from build123d import *

# Parameters (mm, degrees)
EXTRUDE_THIN1_DEPTH   = 6
FILLET1_RADIUS        = 3
FILLET1_LENGTH        = 0.5
F_2_0MM_DOWEL_HOLE1_D = 2


with BuildPart() as part:
    # Sketch1 → Extrude-Thin1 (new body)
    with BuildSketch(Plane.XY):
        Polygon((0, 0), (-6, 0), (-36, 2), (-47.132818026, -3), (-47.337667505, -2.543889606), (-36.091128385, 2.507185105), (-5.983351811, 0.5), (0, 0.5), align=None)
    extrude(amount=EXTRUDE_THIN1_DEPTH)

    # Fillet1: full round fillet: the end face becomes a half cylinder, R = half its width
    fillet1_face = Plane((0, 0.25, 3), x_dir=(0, -1, 0), z_dir=(1, 0, 0))  # on the end face: x along it, z out of the body
    fillet1_slab = fillet1_face.offset(-FILLET1_RADIUS / 2) * Box(FILLET1_LENGTH, 2 * FILLET1_RADIUS, FILLET1_RADIUS, mode=Mode.PRIVATE)  # the body's end, R deep
    fillet1_round = Plane((-3, 0.25, 3), x_dir=(1, 0, 0), z_dir=(0, -1, 0)) * Cylinder(FILLET1_RADIUS, FILLET1_LENGTH, mode=Mode.PRIVATE)  # its axis R under the face
    add(fillet1_slab - fillet1_round, mode=Mode.SUBTRACT)

    # Ø2.0mm Dowel Hole1 (through all)
    with Locations(Plane(origin=(0, 0.5, 0), x_dir=(1, 0, 0), z_dir=(0, 1, 0))):
        with Locations((-3, -3)):
            Hole(F_2_0MM_DOWEL_HOLE1_D / 2)


solid = part.part
Can you work these out from the model? Positions are in its coordinate system, mm. A direction names the side the tool comes from. Give positions to 0.01 mm unless a question says otherwise; leave off trailing zeros. Write each loop counter-clockwise with the first axis right and the second up, starting at its lowest first coordinate (ties: lowest second). Pieces come first, ordered by that corner, then holes. Notation, with made-up numbers: (87, 16) -> (128, 16) arc R25 cw to (128, 47) -> close; hole circle Ø2 at (89, 4). An arc over 180 degrees is marked (long way). Answer as a JSON object with one key per item and string values. Group by question number.
Item 1: Please list where these lines run through material, in increasing order: line 1 (Z direction, x = -3, y = 0.1); line 2 (Y direction, x = -21, z = 4.95); line 3 (Y direction, x = -15.5, z = 3.4). Write a range as [from, to].
Item 2: We'd pull the mould along X, two halves only. Please class faces 1 (the face through (-41.488, -0.465, 2.958)), 2 (the face through (-41.793, -0.054, 2.958)), 3 (the face through (-21.248, 1.518, 2.958)): +X half, -X half, draft (parallel to the pull), parting line (faces both ways), or undercut.
Item 3: Suppose I cut it at C-C (z = 0.95). Please give me the cut outline in (x, y), plus the area to 3 significant figures.
Item 4: Suppose I cut it at A-A (z = 3). Please give me the cut outline in (x, y), plus the area to 3 significant figures.
Item 5: For faces 4 (the face through (-4.4, 0.5, 3)), 5 (the face through (-25.1, 1.6, 0)), 6 (the face through (-4.3, 0, 3)), 7 (the face through (-21, 1, 3)), which set-ups out of +Z, -Z, +X, -X, +Y, -Y let a thin tool reach every point of the face, with its end or its side?
Item 6: I'm going to push flat-ended pins straight in: P1, Ø1, axis at x = -26.5, z = 2.5, coming from the -Y side; P2, Ø1.5, axis at x = -41, z = 5, coming from the +Y side; P3, Ø2, axis at x = -18, z = 2.5, coming from the -Y side. Where does each tip first touch, or does it pass through?
Item 7: Suppose I cut it at B-B (x = -21). Please give me the cut outline in (y, z), plus the area to 3 significant figures.
Item 8: Suppose I cut it at D-D (y = -1.95). Please give me the cut outline in (x, z), plus the area to 3 significant figures.
Findings:
{
 "1": {"line 1": "z = [0, 2], [4, 6]", "line 2": "y = [1, 1.5]", "line 3": "y = [0.63, 1.13]"},
 "2": {"face 1": "undercut", "face 2": "-X half", "face 3": "+X half"},
 "3": {"outline": "(-47.34, -2.54) -> (-47.13, -3) -> (-36, 2) -> (-6, 0) -> (-0.81, 0) -> (-0.81, 0.5) -> (-5.98, 0.5) -> (-36.09, 2.51) -> close", "area": "23.8 mm²"},
 "4": {"outline": "(-47.34, -2.54) -> (-47.13, -3) -> (-36, 2) -> (-6, 0) -> (-4, 0) -> (-4, 0.5) -> (-5.98, 0.5) -> (-36.09, 2.51) -> close; (-2, 0) -> (0, 0) -> (0, 0.5) -> (-2, 0.5) -> close", "area": "23.2 mm²"},
 "5": {"face 4": "+Z, -Z, +X, +Y", "face 5": "-Z, +X, -X, +Y, -Y", "face 6": "+Z, -Z, +X, -Y", "face 7": "+Z, -Z, -Y"},
 "6": {"P1": "stops at y = 1.33", "P2": "stops at y = 0.64", "P3": "stops at y = 0.73"},
 "7": {"outline": "(1, 0) -> (1.5, 0) -> (1.5, 6) -> (1, 6) -> close", "area": "3.01 mm²"},
 "8": {"outline": "(-46.02, 0) -> (-44.79, 0) -> (-44.79, 6) -> (-46.02, 6) -> close", "area": "7.32 mm²"}
}
